Part model, mm, in its own coordinate system. Face numbers are marked on the shaded views. A direction names the side the tool comes from. Coordinates: 2 decimals unless noted, no trailing zeros. Order: outer loops, then holes, each group sorted by start corner. A loop starts at its lowest first (then second) coordinate and runs counter-clockwise, first axis right, second up. Notation, with made-up numbers: M 59.5,-11.75 L 112.5,-11.75 A19 cw 112.5,11.25 Z; hole C 67,-31 d5. An arc over 180 degrees is marked long. Write item = value, one per line. Start each with the question number.
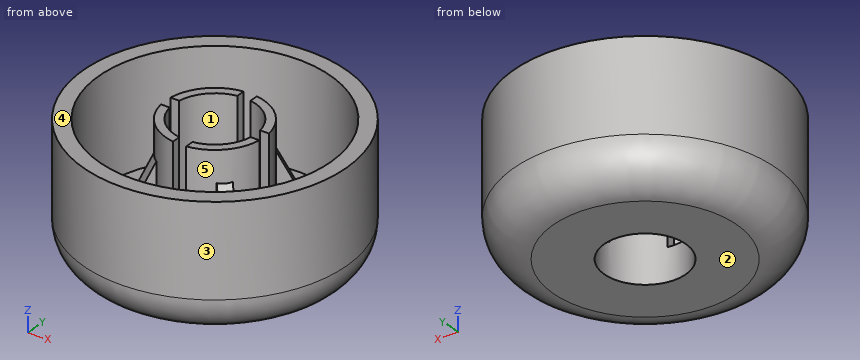
from build123d import *

# Parameters (mm, degrees)
F0_R         = 10
F0_R_2       = 3.1
F1_DEPTH     = 10
F2_R         = 8.8088832383
F2_R_2       = 3.75
F3_DEPTH     = 8
F4_W         = 1
F4_H         = 3.2863240922
F4_W_2       = 2.5055953301
F4_H_2       = 1
F5_DEPTH     = 7.5
F6_R         = 3
F8_DEPTH     = 6
F9_T4_DEPTH  = 1
F9_S5_R      = 3.75
F9_T6_DEPTH  = 5
F9_T10_DEPTH = 1
F9_S11_R     = 3.75
F9_T12_DEPTH = 5
F9_T16_DEPTH = 1
F9_S17_R     = 3.75
F9_T18_DEPTH = 5
F9_T22_DEPTH = 1
F9_S23_R     = 3.75
F9_T24_DEPTH = 5


# Not quite as in the source:
# - a fillet or chamfer that OpenCascade refuses, or shapes differently, is made with other operations: its cross-section is extruded or revolved along the edge and cut away or added
# - two fillets or chamfers of one size are made in one step


with BuildPart() as f1:
    # F0 (on Top) → F1 (new body)
    with BuildSketch(Plane.XY):
        Circle(F0_R)
        Circle(F0_R_2, mode=Mode.SUBTRACT)
    extrude(amount=F1_DEPTH)

    # F2 (on face) → F3 (cut)
    with BuildSketch(Plane.XY.offset(10)):
        Circle(F2_R)
        Circle(F2_R_2, mode=Mode.SUBTRACT)
    extrude(amount=-F3_DEPTH, mode=Mode.SUBTRACT)

    # F4 (on face) → F5 (cut)
    with BuildSketch(Plane.XY.offset(10)):
        Polygon((-2.7353764913, 0.5), (-4.8153767841, 0.5), (-4.8553765493, -0.5), (-2.7353764913, -0.5), align=None)
        Polygon((-0.5, 4.8884870484), (-0.5, 4.6887658536), (-0.5, 1.9834490959), (0.5, 1.9834490959), (0.5, 4.8884870484), align=None)
        with Locations((0, -3.2546973671)):
            Rectangle(F4_W, F4_H)
        with Locations((3.5874212626, 0)):
            Rectangle(F4_W_2, F4_H_2)
    extrude(amount=-F5_DEPTH, mode=Mode.SUBTRACT)

    # F6
    f6_edges = [f1.edges().sort_by_distance(p)[0] for p in [
        (-10, 0, 0),
    ]]
    fillet(f6_edges, radius=F6_R)

    # F7 (on face) → F8 (join)
    with BuildSketch(Plane.XY.offset(2)):
        Polygon((-4.9753358018, 4.2682290206), (-2.9815278958, 2.2744211146), (-2.2744211146, 2.9815278958), (-4.2682290206, 4.9753358018), align=None)
        Polygon((2.2744211146, 2.9815278958), (2.9815278958, 2.2744211146), (4.9753358018, 4.2682290206), (4.2682290206, 4.9753358018), align=None)
        Polygon((-2.2744211146, -2.9815278958), (-2.9815278958, -2.2744211146), (-4.9753358018, -4.2682290206), (-4.2682290206, -4.9753358018), align=None)
        Polygon((2.9815278958, -2.2744211146), (2.2744211146, -2.9815278958), (4.2682290206, -4.9753358018), (4.9753358018, -4.2682290206), align=None)
    extrude(amount=F8_DEPTH)

    # F9: chamfer of 6 x 3 on 4 edges, made by hand


with BuildPart() as f9_tool2:
    # F9_s3 → F9_t4 (new body)
    with BuildSketch(Plane(origin=(0.3535533906, 0.3535533906, 0), x_dir=(0, 0, 1), z_dir=(-0.7071067812, -0.7071067812, 0))):
        Polygon((2, 6.5361873683), (8, 3.5361873683), (8, 6.5361873683), align=None)
    extrude(amount=F9_T4_DEPTH)

    # F9_s5 → F9_t6 (cut, symmetric)
    with BuildSketch(Plane.XY.offset(5)):
        Circle(F9_S5_R)
    extrude(amount=F9_T6_DEPTH, both=True, mode=Mode.SUBTRACT)


with BuildPart() as f1_1:
    add(f1.part)

    # F9_t1: cut F9_tool2
    add(f9_tool2.part, mode=Mode.SUBTRACT)


with BuildPart() as f9_tool8:
    # F9_s9 → F9_t10 (new body)
    with BuildSketch(Plane(origin=(-0.3535533906, -0.3535533906, 0), x_dir=(0, 0, 1), z_dir=(0.7071067812, 0.7071067812, 0))):
        Polygon((2, 6.5361873683), (8, 3.5361873683), (8, 6.5361873683), align=None)
    extrude(amount=F9_T10_DEPTH)

    # F9_s11 → F9_t12 (cut, symmetric)
    with BuildSketch(Plane.XY.offset(5)):
        Circle(F9_S11_R)
    extrude(amount=F9_T12_DEPTH, both=True, mode=Mode.SUBTRACT)


with BuildPart() as f1_2:
    add(f1_1.part)

    # F9_t7: cut F9_tool8
    add(f9_tool8.part, mode=Mode.SUBTRACT)


with BuildPart() as f9_tool14:
    # F9_s15 → F9_t16 (new body)
    with BuildSketch(Plane(origin=(0.3535533906, -0.3535533906, 0), x_dir=(0, 0, 1), z_dir=(-0.7071067812, 0.7071067812, 0))):
        Polygon((2, 6.5361873683), (8, 3.5361873683), (8, 6.5361873683), align=None)
    extrude(amount=F9_T16_DEPTH)

    # F9_s17 → F9_t18 (cut, symmetric)
    with BuildSketch(Plane.XY.offset(5)):
        Circle(F9_S17_R)
    extrude(amount=F9_T18_DEPTH, both=True, mode=Mode.SUBTRACT)


with BuildPart() as f1_3:
    add(f1_2.part)

    # F9_t13: cut F9_tool14
    add(f9_tool14.part, mode=Mode.SUBTRACT)


with BuildPart() as f9_tool20:
    # F9_s21 → F9_t22 (new body)
    with BuildSketch(Plane(origin=(-0.3535533906, 0.3535533906, 0), x_dir=(0, 0, 1), z_dir=(0.7071067812, -0.7071067812, 0))):
        Polygon((2, 6.5361873683), (8, 3.5361873683), (8, 6.5361873683), align=None)
    extrude(amount=F9_T22_DEPTH)

    # F9_s23 → F9_t24 (cut, symmetric)
    with BuildSketch(Plane.XY.offset(5)):
        Circle(F9_S23_R)
    extrude(amount=F9_T24_DEPTH, both=True, mode=Mode.SUBTRACT)


with BuildPart() as f1_4:
    add(f1_3.part)

    # F9_t19: cut F9_tool20
    add(f9_tool20.part, mode=Mode.SUBTRACT)


solid = f1_4.part
Item 1: Cut at D-D, the plane z = 5. Count the separate pieces of the cut face and the enclosed holes in it, and give its area (3 significant figures).
Item 2: Flat gauge pins, fed straight in: pin 1 (0.7 mm diameter, centred on x = -3.5, z = 6.5, fed in from -Y); pin 2 (5 mm diameter, centred on x = 6, z = 4.5, fed in from -Y); pin 3 (0.6 mm diameter, centred on x = 0, y = 3.5, fed in from +Z). Where does each tip first touch, or does it go through?
Item 3: Pull direction Y, two halves, no side cores. Call the marked faces 1, 2 and 3: pulls with the +Y half, pulls with the -Y half, needs draft (parallel to the pull), parting line crosses it, or undercut.
Item 4: Cut at A-A, the plane z = 8.25. Write the cut outline in (x, y), and give its area (3 significant figures).
Item 5: Wall check: line 1 along X through (y, z) = (0.25, 8); line 2 along Y through (x, z) = (1.75, 7.75). Give the ranges that are in metal, low to high. Write a range as [from, to].
Item 6: 3-axis set-ups, long thin cutter, end or side, ignore diameter. For the marked faces 4 and 5: which of +Z, -Z, +X, -X, +Y, -Y reach the whole face in a straight line?
Item 7: Cut at B-B, the plane x = 0. Write the cut outline in (y, z), and give its area (3 significant figures).
Filled sheet:
q1.separate_pieces = 5
q1.enclosed_holes = 1
q1.area = 87.0 mm2
q2.pin_1 = -9.49
q2.pin_2 = -9.37
q2.pin_3 = 2.5
q3.face_1 = undercut
q3.face_2 = needs draft
q3.face_3 = parting line crosses it
q4.outline = C 0,0 d20; M -3.72,-0.5 A3.75 ccw -0.5,-3.72 L -0.5,-3.06 A3.1 cw -3.06,-0.5 Z; M -3.72,0.5 L -3.06,0.5 A3.1 cw -0.5,3.06 L -0.5,3.72 A3.75 ccw Z; M 0.5,-3.72 A3.75 ccw 3.72,-0.5 L 3.06,-0.5 A3.1 cw 0.5,-3.06 Z; M 0.5,3.06 A3.1 cw 3.06,0.5 L 3.72,0.5 A3.75 ccw 0.5,3.72 Z; hole C 0,0 d17.62
q4.area = 81.8 mm2
q5.line_1 = [-10, -8.81], [8.81, 10]
q5.line_2 = [-9.85, -8.63], [-3.32, -2.56], [2.56, 3.32], [8.63, 9.85]
q6.face_4 = +Z, +X, -X, +Y, -Y
q6.face_5 = +Z
q7.outline = M -10,3 A3 ccw -7,0 L -3.1,0 L -3.1,2.5 L -3.75,2.5 L -3.75,2 L -8.81,2 L -8.81,10 L -10,10 Z; M 3.1,0 L 7,0 A3 ccw 10,3 L 10,10 L 8.81,10 L 8.81,2 L 3.75,2 L 3.75,2.5 L 3.1,2.5 Z
q7.area = 43.4 mm2
